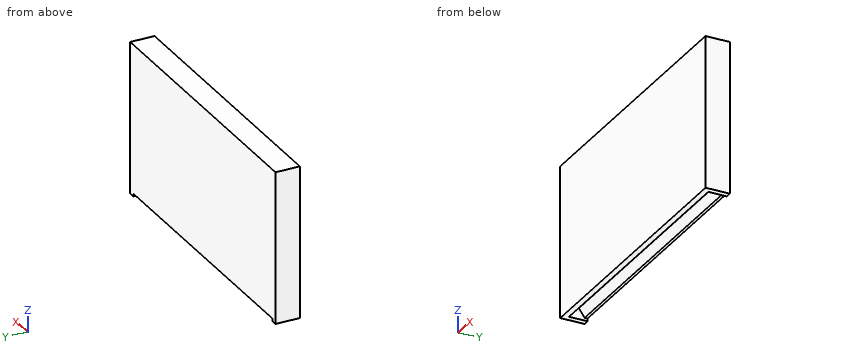
```python
from build123d import *

# Parameters (mm, degrees)
SKETCH1_W           = 240
SKETCH1_H           = 351.15
BOSS_EXTRUDE3_DEPTH = 21
SKETCH5_W           = 248.975913499
SKETCH5_H           = 113.170869772
CUT_EXTRUDE5_DEPTH  = 254
CAVITY1_START       = -93.176553254
CAVITY1_DEPTH       = 230
SKETCH6_W           = 230
SKETCH6_H           = 2.384694545
CUT_EXTRUDE6_DEPTH  = 10


with BuildPart() as part:
    # Sketch1 → Boss-Extrude3 (new body)
    with BuildSketch(Plane(origin=(0, 0, 0), x_dir=(1, 0, 0), z_dir=(0, 1, 0))):
        with Locations((21.823446746, 98.176553254)):
            Rectangle(SKETCH1_W, SKETCH1_H)
    extrude(amount=BOSS_EXTRUDE3_DEPTH)

    # Sketch5 → Cut-Extrude5 (cut)
    with BuildSketch(Plane(origin=(0, 0, -54.481553254), x_dir=(-1, 0, 0), z_dir=(0, 0, -1))):
        with Locations((-20.8478358, 4.110963623)):
            Rectangle(SKETCH5_W, SKETCH5_H)
    extrude(amount=CUT_EXTRUDE5_DEPTH, mode=Mode.SUBTRACT)

    # Cavity1: read off the stored shape, not the designer's step
    # Cavity1 outline → Cavity1 (cut)
    with BuildSketch(Plane.YZ.offset(CAVITY1_START)):
        Polygon((18.5, 60.403141291), (13.5, 67.518446746), (13.5, 67.903141291), (18.5, 67.903141291), (13.5, 75.018446746), (5, 75.018446746), (5, -54.481553254), (13.5, -54.481553254), (13.5, -52.096858709), (18.5, -52.096858709), (13.5, -44.981553254), (13.5, -44.596858709), (18.5, -44.596858709), (13.5, -37.481553254), (13.5, -37.096858709), (18.5, -37.096858709), (13.5, -29.981553254), (13.5, -29.596858709), (18.5, -29.596858709), (13.5, -22.481553254), (13.5, -22.096858709), (18.5, -22.096858709), (13.5, -14.981553254), (13.5, -14.596858709), (18.5, -14.596858709), (13.5, -7.481553254), (13.5, -7.096858709), (18.5, -7.096858709), (13.5, 0.018446746), (13.5, 0.403141291), (18.5, 0.403141291), (13.5, 7.518446746), (13.5, 7.903141291), (18.5, 7.903141291), (13.5, 15.018446746), (13.5, 15.403141291), (18.5, 15.403141291), (13.5, 22.518446746), (13.5, 22.903141291), (18.5, 22.903141291), (13.5, 30.018446746), (13.5, 30.403141291), (18.5, 30.403141291), (13.5, 37.518446746), (13.5, 37.903141291), (18.5, 37.903141291), (13.5, 45.018446746), (13.5, 45.403141291), (18.5, 45.403141291), (13.5, 52.518446746), (13.5, 52.903141291), (18.5, 52.903141291), (13.5, 60.018446746), (13.5, 60.403141291), align=None)
    extrude(amount=CAVITY1_DEPTH, mode=Mode.SUBTRACT)

    # Sketch6 → Cut-Extrude6 (cut)
    with BuildSketch(Plane(origin=(0, 13.5, 0), x_dir=(-1, 0, 0), z_dir=(0, -1, 0))):
        with Locations((-21.823446746, 53.289205982)):
            Rectangle(SKETCH6_W, SKETCH6_H)
    extrude(amount=-CUT_EXTRUDE6_DEPTH, mode=Mode.SUBTRACT)


solid = part.part
```
Read the model definition and answer for the solid it produces. Units are mm, in the model's axes. Coordinates: 2 decimals unless noted, no trailing zeros. Loops run counter-clockwise (first coordinate to the right, second up) from the corner with the lowest first, then second, coordinate; pieces in that order, holes last. Notation, with made-up numbers: (53, 12.5) - (63, 12.5) arc R30 ccw to (63, 41.5) - close; hole circle Ø4 at (69.5, 30.5). An arc over 180 degrees is marked (long way). Answer in a Markdown table with one row per item.
1. Find section A-A, the plane z = -19. Write down the section's boundary in (x, y).
Conclusion:
| item | result |
|---|---|
| outline | (-98.18, 0) - (141.82, 0) - (141.82, 21) - (-98.18, 21) - close; hole (-93.18, 5) - (136.82, 5) - (136.82, 16.32) - (-93.18, 16.32) - close |
2. Straight lines are drawn through the part: line 1 (X direction, y = 11.25, z = -17); line 2 (Z direction, x = -46, y = 9.75); line 3 (Y direction, x = 125, z = -44). For each, find the intervals that lie inside material, in ascending order.
Conclusion:
| item | result |
|---|---|
| line 1 | x = -98.18 to -93.18, 136.82 to 141.82 |
| line 2 | z = 75.02 to 77.4 |
| line 3 | y = 0 to 5, 18.08 to 21 |
3. Given pin 1 (0.8 mm diameter, centred on x = 62.5, y = 19.5, fed in from -Z); pin 2 (3 mm diameter, centred on x = 0.5, y = 9.5, fed in from -Z); pin 3 (4 mm diameter, centred on x = 60, y = 13.5, fed in from -Z), each flat-ended and moving along its own axis, determine where each tip first touches the part or whether it passes through.
Conclusion:
| item | result |
|---|---|
| pin 1 | stops at z = -52.1 |
| pin 2 | stops at z = 75.02 |
| pin 3 | stops at z = -47.83 |
